```python
from build123d import *

# Parameters (mm, degrees)
F0_W     = 119
F0_H     = 80
F1_DEPTH = 1.5
F2_R     = 5
F3_W     = 119
F3_H     = 1.5
F4_DEPTH = 28
F5_R     = 5


with BuildPart() as f1:
    # F0 (on Top) → F1 (new body)
    with BuildSketch(Plane.XY):
        with Locations((-26.13307, -3.521777)):
            Rectangle(F0_W, F0_H)
    extrude(amount=F1_DEPTH)

    # F2
    f2_edges = [f1.edges().sort_by_distance(p)[0] for p in [
        (33.36693, -43.521777, 0.75),
        (33.36693, 36.478223, 0.75),
        (-85.63307, 36.478223, 0.75),
        (-85.63307, -43.521777, 0.75),
    ]]
    fillet(f2_edges, radius=F2_R)

    # F3 (on face) → F4 (join)
    with BuildSketch(Plane.XY.offset(1.5)):
        with Locations((-26.13307, -7.771777)):
            Rectangle(F3_W, F3_H)
    extrude(amount=F4_DEPTH)

    # F5
    f5_edges = [f1.edges().sort_by_distance(p)[0] for p in [
        (-26.13307, -7.021777, 1.5),
        (-26.13307, -8.521777, 1.5),
    ]]
    fillet(f5_edges, radius=F5_R)


solid = f1.part
```
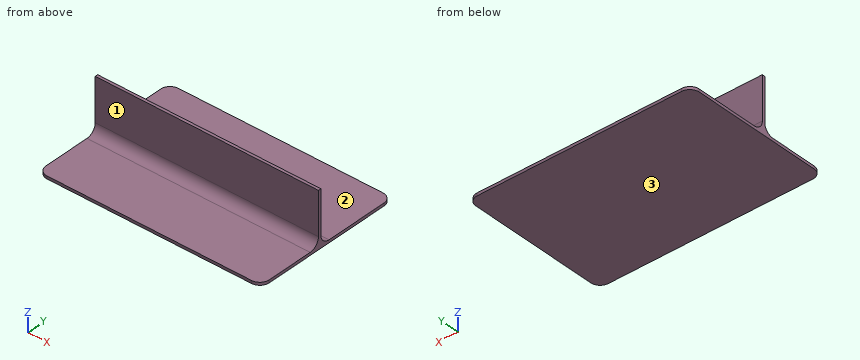
Design review of the part built by this model. Coordinates are the model's own, in mm. Face numbers are marked on the shaded views. A direction names the side the tool comes from. Give positions to 0.01 mm unless a question says otherwise; leave off trailing zeros. Order: outer loops, then holes, each group sorted by start corner. A loop starts at its lowest first (then second) coordinate and runs counter-clockwise, first axis right, second up. Notation, with made-up numbers: (48.25, -14) -> (63.25, -14) arc R23 ccw to (63.25, 15) -> close; hole circle Ø6 at (55, 58). An arc over 180 degrees is marked (long way). Write each question's results on one line, items separated by ' | '. Start each with the question number.
Q1. Add section A-A on x = -33.5. Give the boundary of the cut face in (y, z), and give its area (3 significant figures).
Q2. For pin 1 (10 mm diameter, centred on x = -43, z = 10.5, fed in from +Y); pin 2 (12 mm diameter, centred on x = -50, z = 18, fed in from +Y); pin 3 (6 mm diameter, centred on x = -41.5, z = 14, fed in from -Y), all flat-tipped, find the tip position at first contact; note any pin that passes through.
Q3. Add section C-C on y = 26. Give the boundary of the cut face in (x, z), and give its area (4 significant figures).
Q4. Add section B-B on z = 12.5. Give the boundary of the cut face in (x, y).
Q5. Machinability: for the marked faces 1, 2 and 3, which of the approach directions +Z, -Z, +X, -X, +Y, -Y give a long, thin tool a straight path to every point of the face, cutting with its end or side? Answer none if there is none.
Q6. Wall thickness on L1, parallel to Y at x = -63, z = 21.5; L2, parallel to Z at x = -22, y = 31; L3, parallel to Y at x = 10, z = 2: over which ranges is each line inside the solid? List them lowest first. Write a range as from..to.
Found:
1) outline: (-43.52, 0) -> (36.48, 0) -> (36.48, 1.5) -> (-2.02, 1.5) arc R5 cw to (-7.02, 6.5) -> (-7.02, 29.5) -> (-8.52, 29.5) -> (-8.52, 6.5) arc R5 cw to (-13.52, 1.5) -> (-43.52, 1.5) -> close | area: 173 mm2
2) pin 1: stops at y = -6.92 | pin 2: stops at y = -7.02 | pin 3: stops at y = -8.52
3) outline: (-85.63, 0) -> (33.37, 0) -> (33.37, 1.5) -> (-85.63, 1.5) -> close | area: 178.5 mm2
4) outline: (-85.63, -8.52) -> (33.37, -8.52) -> (33.37, -7.02) -> (-85.63, -7.02) -> close
5) face 1: +Z, +X, -X, -Y | face 2: +Z, +X, -X, +Y | face 3: -Z, +X, -X, +Y, -Y
6) L1: y = -8.52..-7.02 | L2: z = 0..1.5 | L3: y = -11.34..-4.2
